Autodesk Inventor part; units mm, degrees
ref_plane "YZ Plane" through (0, 0, 0) normal (1, 0, 0) x (0, 1, 0)
ref_plane "XZ Plane" through (0, 0, 0) normal (0, 1, 0) x (-1, 0, 0)
ref_plane "XY Plane" through (0, 0, 0) normal (0, 0, 1) x (1, 0, 0)
sketch "Sketch1" plane through (0, 0, 0) normal (1, 0, 0) x (0, 1, 0)
  line L0 (11.2, 0) -> (11.2, -7.3)
  line L1 (11.2, -7.3) -> (0, -7.3)
  line L2 (9.7, 0) -> (9.7, -3.8)
  line L3 (7.7, -5.8) -> (0, -5.8)
  arc A0 (7.7, -5.8) -> (9.7, -3.8) centre (7.7, -3.8) ccw
  line L4 (0, -5.8) -> (0, -7.3)
  line L5 (0, 0) -> (11.2, 0) construction
  line L6 (11.2, 0) -> (11.2, 7.3)
  line L7 (11.2, 7.3) -> (0, 7.3)
  line L8 (9.7, 0) -> (9.7, 3.8)
  line L9 (7.7, 5.8) -> (0, 5.8)
  arc A1 (9.7, 3.8) -> (7.7, 5.8) centre (7.7, 3.8) ccw
  line L10 (0, 5.8) -> (0, 7.3)
  dimension "d2" = 5.8
  dimension "d4" = 1.5
  dimension "d5" = 2
  dimension "d6" = 11.2
  dimension "d7" = 1.5
extrude "Extrusion1" add sketch "Sketch1" along normal blind 11.4
sketch "Sketch3" plane through (0, 0, 0) normal (0, 1, 0) x (-1, 0, 0)
  line L0 (0, -7.3) -> (0, 7.3)
  line L1 (0, -7.3) -> (0, -8.8)
  line L2 (-8.4, -8.8) -> (-8.4, -7.3)
  line L3 (0, -7.3) -> (-11.4, -7.3)
  line L4 (0, -8.8) -> (-8.4, -8.8) construction
  arc A0 (-8.4, -8.8) -> (0, -8.8) centre (-4.2, -8.8) ccw
  circle A1 centre (-4.2, -8.8) radius 1.2
  point P0 (0, 0)
  dimension "d12" = 1.5
  dimension "d13" = 4.2
  dimension "d16" = 2.4
extrude "Extrusion2" add sketch "Sketch3" along normal blind 3.2
mirror "Mirror1" about plane through (0, 0, 0) normal (0, 0, 1) of "Extrusion2"
properties part number "soporteMotor"
For this review, take the finished solid that the model builds, in its own axes (mm). A direction names the side the tool comes from. Give positions to 0.01 mm unless a question says otherwise; leave off trailing zeros. Loops run counter-clockwise (first coordinate to the right, second up) from the corner with the lowest first, then second, coordinate; pieces in that order, holes last. Notation, with made-up numbers: M 43.5,9.25 L 65.5,9.25 A16 ccw 65.5,31.25 Z; hole C -21,-25.5 d2. An arc over 180 degrees is marked long. Answer as a JSON object with one key per item and string values. Group by question number.
Q1. Add section B-B on x = 4.2. Give the boundary of the cut face in (y, z), and give its area (3 significant figures).
Q2. Mouldability with a two-part tool opening along Z and no side actions: class faces 4 (the flat face through (8.4, 2, 8)), 5 (the cylindrical face through (4.1, 1.6, -13)), 6 (the cylindrical face through (4.36, 1.58, -9.99)) as +Z half, -Z half, draft (parallel to the pull), parting line (faces both ways), or undercut.
Q3. Tool access review of faces 1 (the flat face through (6, 9.7, 0)), 2 (the flat face through (4, 3.2, -11)), 3 (the flat face through (8.4, 2, -8)): name each direction out of +Z, -Z, +X, -X, +Y, -Y from which nothing blocks a thin tool from reaching the whole face with its end or side.
Q4. Add section C-C on z = 9.75. Give the boundary of the cut face in (x, y).
Q5. Insertion check: P1, Ø0.8, axis at y = 1, z = -8, coming from the +X side; P2, Ø1.7, axis at x = 3, z = 10, coming from the +Y side; P3, Ø2.5, axis at x = 3.5, z = 1.5, coming from the -Y side. Each pin has a flat end and moves straight along its axis. Give the tip position at first contact, or say it passes through.
Q6. Add section A-A on y = 2. Give the boundary of the cut face in (x, z).
Q7. Add section D-D on y = 7.25. Give the boundary of the cut face in (x, z), and give its area (3 significant figures).
Q8. For probe 1 along Z at (x, y) = (4.2, 1.55); probe 2 along X at (y, z) = (2.4, 8.8); probe 3 along Z at (x, y) = (5, 6.75), list the stretches that pass through material, from the lowest coordinate up. Write a range as [from, to].
Checked values:
{
 "1": {"outline": "M 0,-13 L 3.2,-13 L 3.2,-10 L 0,-10 Z; M 0,-7.6 L 3.2,-7.6 L 3.2,-7.3 L 11.2,-7.3 L 11.2,7.3 L 3.2,7.3 L 3.2,7.6 L 0,7.6 L 0,5.8 L 7.7,5.8 A2 cw 9.7,3.8 L 9.7,-3.8 A2 cw 7.7,-5.8 L 0,-5.8 Z; M 0,10 L 3.2,10 L 3.2,13 L 0,13 Z", "area": "73.8 mm²"},
 "2": {"face 4": "draft", "face 5": "-Z half", "face 6": "undercut"},
 "3": {"face 1": "+X, -X, -Y", "face 2": "-Z, +X, -X, +Y", "face 3": "-Z, +X, +Y, -Y"},
 "4": {"outline": "M 0.11,0 L 3.47,0 L 3.47,3.2 L 0.11,3.2 Z; M 4.93,0 L 8.29,0 L 8.29,3.2 L 4.93,3.2 Z"},
 "5": {"P1": "x = 8.4", "P2": "y = 3.2", "P3": "y = 9.7"},
 "6": {"outline": "M 0,-8.8 A4.2 ccw 8.4,-8.8 L 8.4,-7.3 L 11.4,-7.3 L 11.4,-5.8 L 0,-5.8 Z; M 0,5.8 L 11.4,5.8 L 11.4,7.3 L 8.4,7.3 L 8.4,8.8 A4.2 ccw 0,8.8 Z; hole C 4.2,-8.8 d2.4; hole C 4.2,8.8 d2.4"},
 "7": {"outline": "M 0,-7.3 L 11.4,-7.3 L 11.4,-5.8 L 0,-5.8 Z; M 0,5.8 L 11.4,5.8 L 11.4,7.3 L 0,7.3 Z", "area": "34.2 mm²"},
 "8": {"probe 1": "[-13, -10], [-7.6, -5.8], [5.8, 7.6], [10, 13]", "probe 2": "[0, 3], [5.4, 8.4]", "probe 3": "[-7.3, -5.8], [5.8, 7.3]"}
}
